Here's the drawing with two shaded views (mm, measured from the low corner). I have some questions. A direction names the side the tool comes from. Round coordinates to 2 decimals unless told otherwise and drop trailing zeros. Order: outer loops, then holes, each group sorted by start corner. A loop starts at its lowest first (then second) coordinate and runs counter-clockwise, first axis right, second up. Notation, with made-up numbers: M 19.25,-25.5 L 68.25,-25.5 A25 cw 68.25,-9.5 Z; hole C 78,16 d5. An arc over 180 degrees is marked long. One line per question, with ' | ' between items.
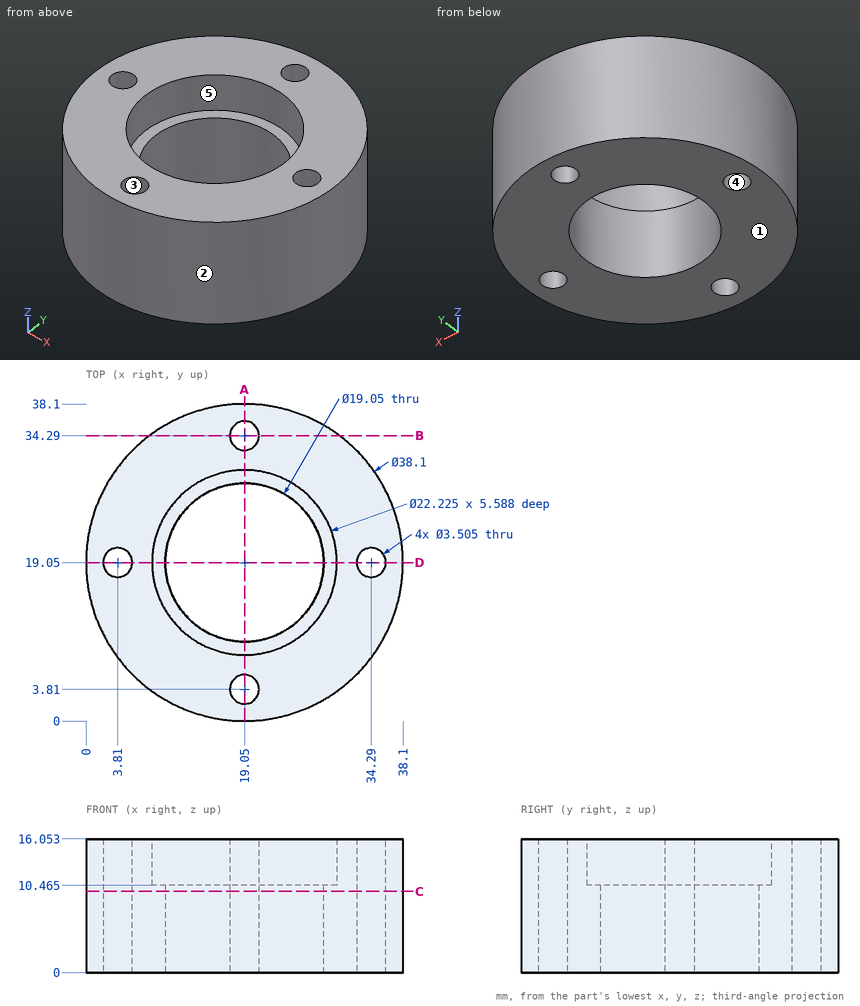
(1) If we section it at B-B on y = 34.29: Please give me the cut outline in (x, z), plus the area to 3 significant figures.
Final values:
outline: M 7.62,0 L 17.3,0 L 17.3,16.05 L 7.62,16.05 Z; M 20.8,0 L 30.48,0 L 30.48,16.05 L 20.8,16.05 Z | area: 311 mm^2
(2) On a 3-axis mill with a long thin cutter (end or side, diameter ignored), from which of +Z, -Z, +X, -X, +Y, -Y can I reach the whole of each face in a straight line? I mean the marked faces 4 and 5. Say none if no direction works.
Final values:
face 4: +Z, -Z | face 5: +Z
(3) If we section it at A-A on x = 19.05: Please give me the cut outline in (y, z) (1 decimal).
Final values:
outline: M 0,0 L 2.1,0 L 2.1,16.1 L 0,16.1 Z; M 5.6,0 L 9.5,0 L 9.5,10.5 L 7.9,10.5 L 7.9,16.1 L 5.6,16.1 Z; M 28.6,0 L 32.5,0 L 32.5,16.1 L 30.2,16.1 L 30.2,10.5 L 28.6,10.5 Z; M 36,0 L 38.1,0 L 38.1,16.1 L 36,16.1 Z
(4) Will these pins go through, and if not, where does the flat tip stop? pin 1 Ø4 at (x, y) = (19.05, 34.29) entering from -Z; pin 2 Ø15 at (x, y) = (19.05, 19.05) entering from -Z; pin 3 Ø3 at (x, z) = (30, 14.5) entering from -Y; pin 4 Ø6 at (x, z) = (13.5, 3) entering from -Y.
Final values:
pin 1: z = 0 | pin 2: through | pin 3: y = 2.51 | pin 4: y = 0.17
(5) If we section it at C-C on z = 9.75: State how many separate pieces and enclosed holes the cut face has.
Final values:
separate pieces: 1 | enclosed holes: 5
(6) Thinking about a two-plate mould opening in Y: for the marked faces 1, 2 and 3, which applies, released by +Y, released by -Y, zero draft, split by the parting line, or undercut?
Final values:
face 1: zero draft | face 2: split by the parting line | face 3: undercut
(7) Please list where these lines run through material, in increasing order: probe 1 along Y at (x, z) = (19.05, 14.35); probe 2 along Y at (x, z) = (19.05, 4.75) (1 decimal); probe 3 along Y at (x, z) = (34.5, 13) (1 decimal). Write a range as [from, to].
Final values:
probe 1: [0, 2.06], [5.56, 7.94], [30.16, 32.54], [36.04, 38.1] | probe 2: [0, 2.1], [5.6, 9.5], [28.6, 32.5], [36, 38.1] | probe 3: [7.9, 17.3], [20.8, 30.2]
